Build history of the part. All positions in model axes, mm. A direction names the side the tool comes from. Round coordinates to 2 decimals unless told otherwise and drop trailing zeros. Write each loop counter-clockwise with the first axis right and the second up, starting at its lowest first coordinate (ties: lowest second). Pieces come first, ordered by that corner, then holes. Notation, with made-up numbers: (-30, 7) -> (-26, 7) arc R26 ccw to (-26, 39) -> close; hole circle Ø5 at (18.5, 46.5). An arc over 180 degrees is marked (long way). Return JSON: item names as keys, results as strings.
from build123d import *

# Parameters (mm, degrees)
EXTRUDE_THIN1_DEPTH = 22
SKETCH4_R           = 0.649105381
SKETCH4_R_2         = 0.65234644
SKETCH4_R_3         = 0.906952967
SKETCH4_W           = 5.036303432
SKETCH4_H           = 5.470796117
CUT_EXTRUDE2_DEPTH  = 38.347454818
SKETCH8_R           = 0.450837693
SKETCH8_R_2         = 0.449707116
SKETCH8_R_3         = 0.445855953
CUT_EXTRUDE5_DEPTH  = 38.347454818
SKETCH9_W           = 17.606045563
SKETCH9_H           = 3.76709992
SKETCH9_H_2         = 4.767878547
CUT_EXTRUDE6_DEPTH  = 38.347454818


with BuildPart() as part:
    # Sketch2 → Extrude-Thin1 (new body)
    with BuildSketch(Plane(origin=(0, 0, 0), x_dir=(1, 0, 0), z_dir=(0, 1, 0))):
        Polygon((0, 0), (0, -21.46884451), (17.606045563, -21.46884451), (17.606045563, -24.512436456), (-3.043591946, -24.512436456), (-3.043591946, 0), align=None)
    extrude(amount=EXTRUDE_THIN1_DEPTH)

    # Sketch4 → Cut-Extrude2 (cut, through all)
    with BuildSketch(Plane(origin=(0, 0, 0), x_dir=(0, 0, -1), z_dir=(1, 0, 0))):
        with Locations((-1.261501122, 10.771672365)):
            Circle(SKETCH4_R)
        with Locations((-20.011001783, 10.771672365)):
            Circle(SKETCH4_R_2)
        with Locations((-10.589323514, 17.938155066)):
            Circle(SKETCH4_R_3)
        with Locations((-10.589323514, 0.943208514)):
            Rectangle(SKETCH4_W, SKETCH4_H)
    extrude(amount=-CUT_EXTRUDE2_DEPTH, mode=Mode.SUBTRACT)

    # Sketch8 → Cut-Extrude5 (cut, through all)
    with BuildSketch(Plane.XY):
        with Locations(Location((3.77269277, 16.868201952, 0), (0, 0, 180))):
            Circle(SKETCH8_R)
        with Locations(Location((12.628067292, 16.868201952, 0), (0, 0, 180))):
            Circle(SKETCH8_R)
        with Locations(Location((13.078904985, 6.223556551, 0), (0, 0, 180))):
            Circle(SKETCH8_R_2)
        with Locations(Location((3.321855077, 6.223556551, 0), (0, 0, 180))):
            Circle(SKETCH8_R_3)
    extrude(amount=CUT_EXTRUDE5_DEPTH, mode=Mode.SUBTRACT)

    # Sketch9 → Cut-Extrude6 (cut, through all)
    with BuildSketch(Plane.XY):
        with Locations((8.803022782, 20.11645004)):
            Rectangle(SKETCH9_W, SKETCH9_H)
        with Locations((8.803022782, 2.383939274)):
            Rectangle(SKETCH9_W, SKETCH9_H_2)
    extrude(amount=CUT_EXTRUDE6_DEPTH, mode=Mode.SUBTRACT)


solid = part.part
Q1. Saw through at A-A on z = 22.5. List the corners of the cut face in (x, y).
Verdict:
{"outline": "(-3.04, 0) -> (0, 0) -> (0, 4.77) -> (17.61, 4.77) -> (17.61, 18.23) -> (0, 18.23) -> (0, 22) -> (-3.04, 22) -> close; hole circle Ø0.89 at (3.32, 6.22); hole circle Ø0.9 at (3.77, 16.87); hole circle Ø0.9 at (12.63, 16.87); hole circle Ø0.9 at (13.08, 6.22)"}
Q2. 3-axis set-ups, long thin cutter, end or side, ignore diameter. For faces 1 (the flat face through (9, 4.768, 23)), 2 (the flat face through (-2, 2, 8.071)), 3 (the flat face through (9, 11, 21.469)), 4 (the flat face through (9, 18.233, 23)): which of +Z, -Z, +X, -X, +Y, -Y reach the whole face in a straight line?
Verdict:
{"face 1": "+Z, -Z, +X, -Y", "face 2": "+X, -X, -Y", "face 3": "-Z, +X, +Y, -Y", "face 4": "+Z, -Z, +X, +Y"}
Q3. Saw through at C-C on x = 14.75. List the corners of the cut face in (y, z), then the cut area to 3 significant figures.
Verdict:
{"outline": "(4.77, 21.47) -> (18.23, 21.47) -> (18.23, 24.51) -> (4.77, 24.51) -> close", "area": "41.0 mm²"}
Q4. Pin check, flat tips, straight feed: pin 1 Ø5 at (x, y) = (10.5, 11.5) entering from -Z; pin 2 Ø1 at (y, z) = (10.77, 1.26) entering from -X; pin 3 Ø0.9 at (x, z) = (-1.5, 10.5) entering from -Y; pin 4 Ø3.5 at (x, z) = (9, 23.5) entering from -Y. Stop position of each tip, or through.
Verdict:
{"pin 1": "stops at z = 21.47", "pin 2": "passes through", "pin 3": "stops at y = 3.68", "pin 4": "stops at y = 4.77"}
Q5. Saw through at D-D on z = 12. List the corners of the cut face in (x, y), then the cut area to 3 significant figures.
Verdict:
{"outline": "(-3.04, 3.68) -> (0, 3.68) -> (0, 22) -> (-3.04, 22) -> close", "area": "55.8 mm²"}
Q6. Saw through at B-B on y = 15.75. List the corners of the cut face in (x, z).
Verdict:
{"outline": "(-3.04, 0) -> (0, 0) -> (0, 21.47) -> (17.61, 21.47) -> (17.61, 24.51) -> (-3.04, 24.51) -> close"}
Q7. Wall check: L1, parallel to Z at x = 6, y = 7; L2, parallel to Y at x = -0.5, z = 8.75; L3, parallel to X at y = 2.25, z = 20.75. Give the ranges that are in metal, low to high.
Verdict:
{"L1": "z = 21.47 to 24.51", "L2": "y = 3.68 to 22", "L3": "x = -3.04 to 0"}
Q8. Two-plate mould, pull along Z, no slides. Class faces 5 (the flat face through (-2, 3.679, 11)), 6 (the cylindrical face through (12.69, 16.42, 22.97)), 7 (the cylindrical face through (-1.5, 17.39, 11.31)), 8 (the flat face through (7, 11, 24.512)): +Z half, -Z half, draft (parallel to the pull), parting line (faces both ways), or undercut.
Verdict:
{"face 5": "undercut", "face 6": "draft", "face 7": "undercut", "face 8": "+Z half"}
